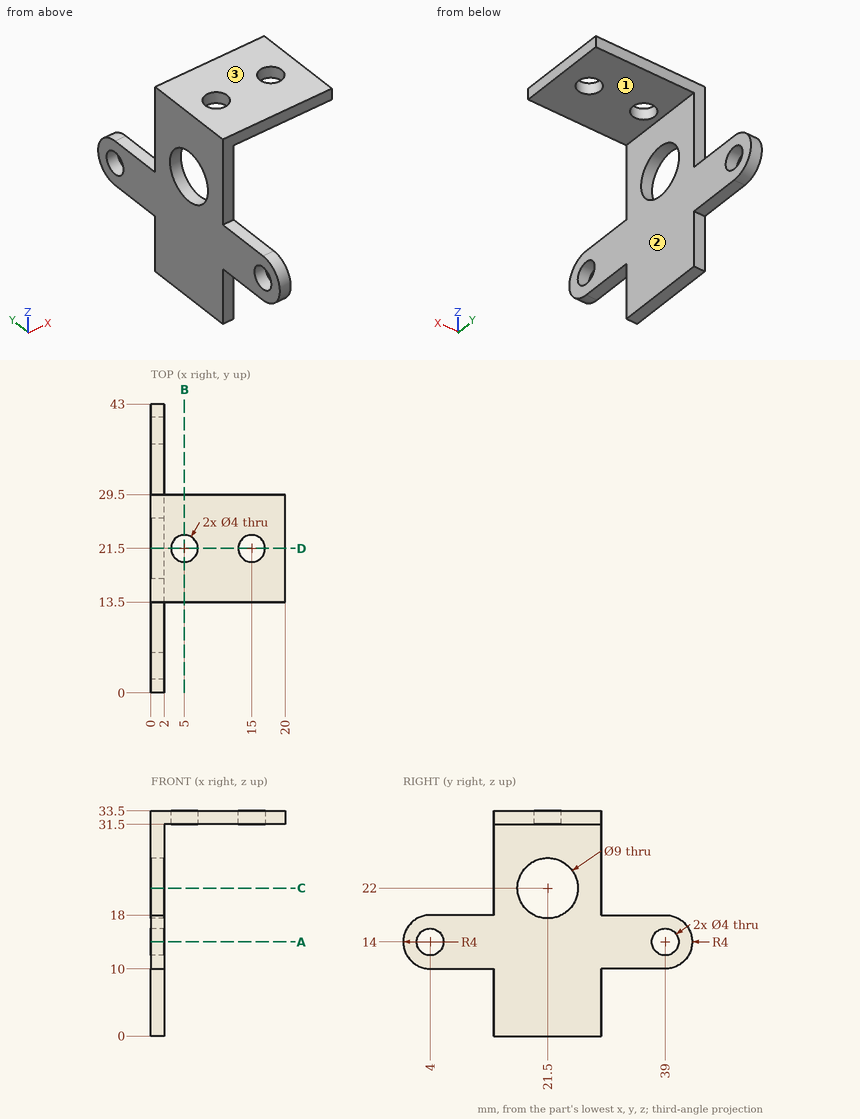
The drawing under review shows one solid part. Ordinate dimensions are in mm from its lowest x, y, z. Coordinates: 2 decimals unless noted, no trailing zeros. Order: outer loops, then holes, each group sorted by start corner. A loop starts at its lowest first (then second) coordinate and runs counter-clockwise, first axis right, second up. Notation, with made-up numbers: M 25.25,42 L 49.25,42 A25 ccw 49.25,73 Z; hole C -27,-21 d5. An arc over 180 degrees is marked long. Use a Markdown table: item, result.
(1) Draft analysis for pull direction Z (two halves, no side actions). For the marked faces 1, 2 and 3, state which applies: released by +Z, released by -Z, zero draft, split by the parting line, or undercut.
Worked answers:
| item | result |
|---|---|
| face 1 | released by -Z |
| face 2 | zero draft |
| face 3 | released by +Z |
(2) Add section C-C (z = 22). Give the boundary of the cut face in (x, y), then the cut area to 3 significant figures.
Worked answers:
| item | result |
|---|---|
| outline | M 0,13.5 L 2,13.5 L 2,17 L 0,17 Z; M 0,26 L 2,26 L 2,29.5 L 0,29.5 Z |
| area | 14.0 mm2 |
(3) For P1, Ø6.5, axis at x = 5, y = 21.5, coming from the -Z side; P2, Ø10, axis at x = 2.5, y = 6.5, coming from the -Z side; P3, Ø11.5, axis at y = 21.5, z = 22, coming from the +X side; P4, Ø0.6, axis at x = 1, y = 34, coming from the +Z side, all flat-tipped, find the tip position at first contact; note any pin that passes through.
Worked answers:
| item | result |
|---|---|
| P1 | stops at z = 0 |
| P2 | stops at z = 10 |
| P3 | stops at x = 2 |
| P4 | stops at z = 18 |
(4) Add section B-B (x = 5). Give the boundary of the cut face in (y, z), then the cut area to 3 significant figures.
Worked answers:
| item | result |
|---|---|
| outline | M 13.5,31.5 L 19.5,31.5 L 19.5,33.5 L 13.5,33.5 Z; M 23.5,31.5 L 29.5,31.5 L 29.5,33.5 L 23.5,33.5 Z |
| area | 24.0 mm2 |
(5) Add section D-D (y = 21.5). Give the boundary of the cut face in (x, z).
Worked answers:
| item | result |
|---|---|
| outline | M 0,0 L 2,0 L 2,17.5 L 0,17.5 Z; M 0,26.5 L 2,26.5 L 2,31.5 L 3,31.5 L 3,33.5 L 0,33.5 Z; M 7,31.5 L 13,31.5 L 13,33.5 L 7,33.5 Z; M 17,31.5 L 20,31.5 L 20,33.5 L 17,33.5 Z |
(6) Wall thickness on probe 1 along Y at (x, z) = (1.5, 14); probe 2 along Y at (x, z) = (15, 32.5); probe 3 along Y at (x, z) = (1.35, 22): over which ranges is each line inside the solid? List them lowest first.
Worked answers:
| item | result |
|---|---|
| probe 1 | y = 0 to 2, 6 to 37, 41 to 43 |
| probe 2 | y = 13.5 to 19.5, 23.5 to 29.5 |
| probe 3 | y = 13.5 to 17, 26 to 29.5 |
(7) Add section A-A (z = 14). Give the boundary of the cut face in (x, y), then the cut area to 3 significant figures.
Worked answers:
| item | result |
|---|---|
| outline | M 0,0 L 2,0 L 2,2 L 0,2 Z; M 0,6 L 2,6 L 2,37 L 0,37 Z; M 0,41 L 2,41 L 2,43 L 0,43 Z |
| area | 70.0 mm2 |
